The model under review builds one solid part; all positions refer to its coordinate system, in mm. A direction names the side the tool comes from. Coordinates: 2 decimals unless noted, no trailing zeros. Write each loop counter-clockwise with the first axis right and the second up, starting at its lowest first coordinate (ties: lowest second). Pieces come first, ordered by that corner, then holes. Notation, with made-up numbers: (82.25, 28.5) - (98.25, 28.5) arc R25 ccw to (98.25, 63.5) - close; hole circle Ø1 at (36, -23). An arc over 180 degrees is marked (long way). Return JSON: item names as keys, results as strings. Group by question number.
(1) To check wall thickness, follow L1, parallel to X at y = -84.5, z = 3.25; L2, parallel to Y at x = 1.5, z = 0.75; L3, parallel to Y at x = -9.5, z = 4. State the ranges of each line that lie inside material, in increasing order. Write a range as from..to.
(2) Tool access review of faces 5 (the face through (26.988, 41, 3)), 6 (the face through (33.338, 136, 3)): name each direction out of +Z, -Z, +X, -X, +Y, -Y from which nothing blocks a thin tool from reaching the whole face with its end or side.
(3) For pin 1 Ø1.9 at (y, z) = (46.5, 3.5) entering from +X; pin 2 Ø3 at (x, z) = (31.5, 4) entering from -Y, all flat-tipped, find the tip position at first contact; note any pin that passes through.
(4) We need section A-A on z = 5.25. State the section outline as (x, y) points, then the cut area to 3 significant figures.
(5) Draft analysis for pull direction Y (two halves, no side actions). For faces 1 (the face through (30, 120.65, 3)), 2 (the face through (30, 57.15, 3)), 3 (the face through (26.988, -86, 3)), 4 (the face through (30, -69.85, 3)), state which applies: released by +Y, released by -Y, zero draft, split by the parting line, or undercut.
(6) We need section C-C on x = 0. State the section outline as (y, z) points, then the cut area to 3 significant figures.
(7) We need section B-B on y = 98.5. State the section outline as (x, z) points, then the cut area to 3 significant figures.
```python
from build123d import *

# Parameters (mm, degrees)
BOSS_EXTRUDE1_DEPTH = 6.35
SKETCH2_W           = 12.7
SKETCH2_H           = 6.35
CUT_EXTRUDE1_DEPTH  = 6.35


with BuildPart() as part:
    # Sketch1 → Boss-Extrude1 (new body)
    with BuildSketch(Plane.XY):
        Polygon((-26.9875, -101.6), (14.2875, -101.6), (14.2875, -107.95), (26.9875, -107.95), (26.9875, -69.85), (33.3375, -69.85), (33.3375, -38.1), (26.9875, -38.1), (26.9875, -6.35), (33.3375, -6.35), (33.3375, 25.4), (26.9875, 25.4), (26.9875, 57.15), (33.3375, 57.15), (33.3375, 88.9), (26.9875, 88.9), (26.9875, 120.65), (33.3375, 120.65), (33.3375, 152.4), (26.9875, 152.4), (-26.9875, 101.6), align=None)
    extrude(amount=BOSS_EXTRUDE1_DEPTH)

    # Sketch2 → Cut-Extrude1 (cut)
    with BuildSketch(Plane(origin=(0, 0, 0), x_dir=(-1, 0, 0), z_dir=(0, 0, -1))):
        with Locations((-20.6375, -104.775)):
            Rectangle(SKETCH2_W, SKETCH2_H)
    extrude(amount=-CUT_EXTRUDE1_DEPTH, mode=Mode.SUBTRACT)


solid = part.part
```
Ans:
{
 "1": {"L1": "-26.99..26.99", "L2": "-101.6..128.41", "L3": "-101.6..118.06"},
 "2": {"face 5": "+Z, -Z, +X", "face 6": "+Z, -Z, +X, +Y, -Y"},
 "3": {"pin 1": "x = 26.99", "pin 2": "y = -69.85"},
 "4": {"outline": "(-26.99, -101.6) - (26.99, -101.6) - (26.99, -69.85) - (33.34, -69.85) - (33.34, -38.1) - (26.99, -38.1) - (26.99, -6.35) - (33.34, -6.35) - (33.34, 25.4) - (26.99, 25.4) - (26.99, 57.15) - (33.34, 57.15) - (33.34, 88.9) - (26.99, 88.9) - (26.99, 120.65) - (33.34, 120.65) - (33.34, 152.4) - (26.99, 152.4) - (-26.99, 101.6) - close", "area": "13,100 mm²"},
 "5": {"face 1": "undercut", "face 2": "undercut", "face 3": "zero draft", "face 4": "released by -Y"},
 "6": {"outline": "(-101.6, 0) - (127, 0) - (127, 6.35) - (-101.6, 6.35) - close", "area": "1,450 mm²"},
 "7": {"outline": "(-26.99, 0) - (26.99, 0) - (26.99, 6.35) - (-26.99, 6.35) - close", "area": "343 mm²"}
}
